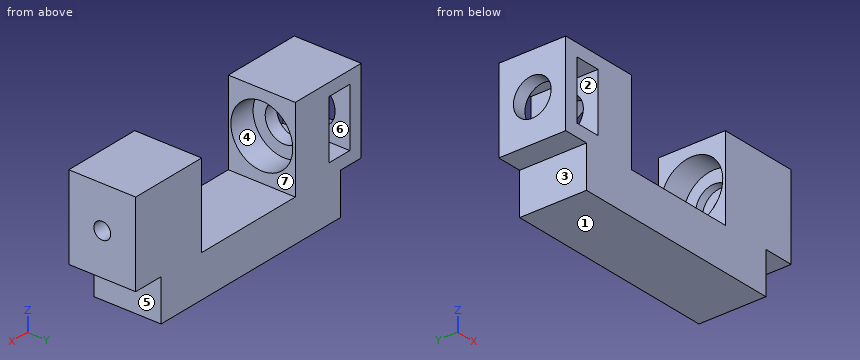
from build123d import *

# Parameters (mm, degrees)
SHAPE_DEPTH                   = 4
SHAPE_DEPTH_BACK              = 4
ESQUISSE19_R                  = 2.25
HOLEAXE_MOTOR_DEPTH           = 13
ESQUISSE20_R                  = 3.7
HOLEBEARING_MOTOR_DEPTH       = 3.2
ESQUISSE21_R                  = 2.2
ENTRETOISEBEARING_MOTOR_DEPTH = 1
EXT_MOTOR_START               = 3
ESQUISSE22_W                  = 10
ESQUISSE22_H                  = 8
ESQUISSE22_R                  = 2.25
EXT_MOTOR_DEPTH               = 3
ESQUISSE23_W                  = 3
ESQUISSE23_H                  = 7
HOLESCREWLESS_MOTOR_DEPTH     = 10
ESQUISSE24_W                  = 10
ESQUISSE24_H                  = 8
BOSS_EXTRU_1_DEPTH            = 3
ESQUISSE25_W                  = 5
ESQUISSE25_H                  = 8
ADJUSTMENT_ATTACH_DEPTH       = 0.65
ESQUISSE26_R                  = 1
REMOVE_HELPER_DEPTH           = 10


with BuildPart() as part:
    # Esquisse17 → Shape (new, two sides: drawn at the far end of the back side and taken through both)
    with BuildSketch(Plane(origin=(0, 40, 0), x_dir=(-1, 0, 0), z_dir=(0, -1, 0)).offset(-SHAPE_DEPTH_BACK)):
        Polygon((13.25, 105), (13.25, 95), (6.75, 95), (6.75, 105), (-6.75, 105), (-6.75, 95), (-13.25, 95), (-13.25, 105), (-13.25, 110), (13.25, 110), align=None)
    extrude(amount=SHAPE_DEPTH + SHAPE_DEPTH_BACK)

    # Esquisse19 → HoleAxe_motor (cut)
    with BuildSketch(Plane.ZY.offset(13.25)):
        with Locations((-100, 40)):
            Circle(ESQUISSE19_R)
    extrude(amount=-HOLEAXE_MOTOR_DEPTH, mode=Mode.SUBTRACT)

    # Esquisse20 → HoleBearing_motor (cut)
    with BuildSketch(Plane.ZY.offset(-6.75)):
        with Locations((-100, 40)):
            Circle(ESQUISSE20_R)
    holebearing_motor = extrude(amount=-HOLEBEARING_MOTOR_DEPTH, mode=Mode.SUBTRACT)

    # Symétrie3: HoleBearing_motor across plane
    add(holebearing_motor.mirror(Plane(origin=(0, 0, 0), x_dir=(0, 0, 1), z_dir=(1, 0, 0))), mode=Mode.SUBTRACT)

    # Esquisse21 → entretoiseBearing_motor (cut)
    with BuildSketch(Plane.ZY.offset(-9.95)):
        with Locations((-100, 40)):
            Circle(ESQUISSE21_R)
    extrude(amount=-ENTRETOISEBEARING_MOTOR_DEPTH, mode=Mode.SUBTRACT)

    # Esquisse22 → Ext_motor (add)
    with BuildSketch(Plane.ZY.offset(13.25).offset(EXT_MOTOR_START)):
        with Locations((-100, 40)):
            Rectangle(ESQUISSE22_W, ESQUISSE22_H)
        with Locations((-100, 40)):
            Circle(ESQUISSE22_R, mode=Mode.SUBTRACT)
    extrude(amount=-EXT_MOTOR_DEPTH)

    # Esquisse23 → HoleScrewLess_motor (cut)
    with BuildSketch(Plane(origin=(0, 44, 0), x_dir=(1, 0, 0), z_dir=(0, 1, 0))):
        with Locations((-13.1, 100)):
            Rectangle(ESQUISSE23_W, ESQUISSE23_H)
    extrude(amount=-HOLESCREWLESS_MOTOR_DEPTH, mode=Mode.SUBTRACT)

    # Esquisse24 → Boss.-Extru.1 (add)
    with BuildSketch(Plane(origin=(13.25, 0, 0), x_dir=(0, 0, -1), z_dir=(1, 0, 0))):
        with Locations((100, 40)):
            Rectangle(ESQUISSE24_W, ESQUISSE24_H)
    extrude(amount=BOSS_EXTRU_1_DEPTH)

    # Esquisse25 → Adjustment attach (cut)
    with BuildSketch(Plane(origin=(13.25, 0, 0), x_dir=(0, 0, -1), z_dir=(1, 0, 0))):
        with Locations((107.5, 40)):
            Rectangle(ESQUISSE25_W, ESQUISSE25_H)
    extrude(amount=-ADJUSTMENT_ATTACH_DEPTH, mode=Mode.SUBTRACT)

    # Esquisse26 → Remove helper (cut)
    with BuildSketch(Plane.ZY.offset(-10.95)):
        with Locations((-100, 40)):
            Circle(ESQUISSE26_R)
    extrude(amount=-REMOVE_HELPER_DEPTH, mode=Mode.SUBTRACT)


solid = part.part
Here's how the part is built. I have some questions about the finished solid (model axes, mm). Face numbers are marked on the shaded views. A direction names the side the tool comes from. Give positions to 0.01 mm unless a question says otherwise; leave off trailing zeros. Order: outer loops, then holes, each group sorted by start corner. A loop starts at its lowest first (then second) coordinate and runs counter-clockwise, first axis right, second up. Notation, with made-up numbers: (46, 89.25) -> (67, 89.25) arc R19 cw to (67, 109.25) -> close; hole circle Ø7 at (19.25, 12.5). An arc over 180 degrees is marked (long way). Use a Markdown table: item, result. Add a question column.
Item 1: Imagine slicing it at A-A on z = -104.5. Please give me the cut outline in (x, y), plus the area to 3 significant figures.
Item 2: If we mould it in two halves opening along X, with no side actions, what happens to the marked faces 1, 2 and 3? For each: pulls with the +X half, pulls with the -X half, needs draft (parallel to the pull), parting line crosses it, or undercut.
Item 3: Imagine slicing it at B-B on x = 8.5. Please give me the cut outline in (y, z), plus the area to 3 significant figures.
Item 4: I need wall thicknesses on line 1 (X direction, y = 37.25, z = -102.75); line 2 (X direction, y = 41.5, z = -97.75); line 3 (Y direction, x = -8.4, z = -100). Which ranges of each line are inside material? Lowest first, please.
Item 5: Imagine slicing it at D-D on z = -100. Give the number of separate pieces and of enclosed holes in the cut face, plus the area to 3 significant figures.
Item 6: Imagine slicing it at C-C on y = 43.25. Please give me the cut outline in (x, z).
Item 7: For the marked faces 4, 5, 6 and 7, which set-ups out of +Z, -Z, +X, -X, +Y, -Y let a thin tool reach every point of the face, with its end or its side?
Item 8: Will these pins go through, and if not, where does the flat tip stop? pin 1 (2 mm diameter, centred on y = 40, z = -99, fed in from -X); pin 2 (1.5 mm diameter, centred on y = 38.5, z = -108.5, fed in from -X); pin 3 (2.5 mm diameter, centred on x = -15.5, y = 40.5, fed in from -Z); pin 4 (1.6 mm diameter, centred on y = 40, z = -100, fed in from +X).
Data:
| question | item | result |
|---|---|---|
| 1 | outline | (-16.25, 36) -> (-6.75, 36) -> (-6.75, 44) -> (-16.25, 44) -> close; (6.75, 36) -> (16.25, 36) -> (16.25, 44) -> (6.75, 44) -> close |
| 1 | area | 152 mm² |
| 2 | face 1 | needs draft |
| 2 | face 2 | undercut |
| 2 | face 3 | pulls with the -X half |
| 3 | outline | (36, -110) -> (44, -110) -> (44, -95) -> (36, -95) -> close; hole circle Ø7.4 at (40, -100) |
| 3 | area | 77.0 mm² |
| 4 | line 1 | x = -16.25 to -14.6, -11.6 to -6.75, 6.75 to 16.25 |
| 4 | line 2 | x = -16.25 to -14.6, -11.6 to -9.95, 9.95 to 16.25 |
| 4 | line 3 | y = 36 to 36.3, 43.7 to 44 |
| 5 | separate pieces | 6 |
| 5 | enclosed holes | 0 |
| 5 | area | 50.8 mm² |
| 6 | outline | (-16.25, -105) -> (-13.25, -105) -> (-13.25, -110) -> (12.6, -110) -> (12.6, -105) -> (16.25, -105) -> (16.25, -95) -> (6.75, -95) -> (6.75, -98.23) -> (9.95, -98.23) -> (9.95, -101.77) -> (6.75, -101.77) -> (6.75, -105) -> (-6.75, -105) -> (-6.75, -101.77) -> (-9.95, -101.77) -> (-9.95, -98.23) -> (-6.75, -98.23) -> (-6.75, -95) -> (-16.25, -95) -> close; hole (-14.6, -103.5) -> (-11.6, -103.5) -> (-11.6, -96.5) -> (-14.6, -96.5) -> close |
| 7 | face 4 | none |
| 7 | face 5 | -Z, +X, +Y, -Y |
| 7 | face 6 | +Y, -Y |
| 7 | face 7 | +Z, +Y, -Y |
| 8 | pin 1 | stops at x = 10.95 |
| 8 | pin 2 | stops at x = -13.25 |
| 8 | pin 3 | stops at z = -105 |
| 8 | pin 4 | passes through |
